Read the model definition and answer for the solid it produces. Units are mm, in the model's axes. A direction names the side the tool comes from. Coordinates: 2 decimals unless noted, no trailing zeros. Loops run counter-clockwise (first coordinate to the right, second up) from the corner with the lowest first, then second, coordinate; pieces in that order, holes last. Notation, with made-up numbers: (38, 83) -> (51, 83) arc R16 cw to (51, 100) -> close; hole circle Ø1 at (87, 54.25). An arc over 180 degrees is marked (long way). Answer as a JSON object with one key per item and string values. Group by question number.
Q1. The part is cut by section D-D on z = 8.5. Write down the section's boundary in (x, y).
Q2. The part is cut by section B-B on x = 12.5. State how many separate pieces and enclosed holes the cut face has, and give its area (3 significant figures).
Q3. Each of these flat-tipped pins is pushed along its axis until it touches: P1, Ø6, axis at y = 2, z = 5, coming from the +X side; P2, Ø1, axis at y = -3.5, z = 1, coming from the +X side; P3, Ø4, axis at x = -7, y = -2.5, coming from the -Z side; P4, Ø3, axis at y = 1.5, z = 1.5, coming from the -X side. Where does it stop, or does it pass through?
Q4. Straight lines are drawn through the part: line 1 along Y through (x, z) = (-13, 4.8); line 2 along Y through (x, z) = (12, 1.25); line 3 along Z through (x, y) = (-8.5, -4). For each, find the intervals that lie inside material, in ascending order. Write a range as [from, to].
Q5. The part is cut by section A-A on z = 5.25. Write down the section's boundary in (x, y), and give its area (3 significant figures).
Q6. Determine the mould class of faces 1 (the flat face through (7.5, 0, 5)), 2 (the cylindrical face through (18, 0, 9)), 3 (the flat face through (-10, 0, 7.5)) for opening direction Z: released by +Z, released by -Z, zero draft, split by the parting line, or undercut.
Q7. For faces 4 (the flat face through (10, 2, 2.2)), 5 (the flat face through (13, 3.05, 1)), 6 (the flat face through (-10, 0, 2.5)), 7 (the flat face through (-7.5, 0, 9)), determine the directions among +Z, -Z, +X, -X, +Y, -Y from which every point of the face is accessible in a straight line to the end or side of a thin tool.
from build123d import *

# Parameters (mm, degrees)
EXTRUDE_1_DEPTH     = 10
SKETCH_3_W          = 10.5
SKETCH_3_H          = 5.6
CUT_EXTRUDE_2_DEPTH = 23.891046285
SKETCH_4_W          = 10.5
SKETCH_4_H          = 2.5
CUT_EXTRUDE_3_DEPTH = 23.891046285
SKETCH_2_R          = 4
CUT_EXTRUDE_4_DEPTH = 3
CUT_EXTRUDE_4_DRAFT = -20
CUT_EXTRUDE_5_DEPTH = 2.5
SKETCH_9_R          = 2
CUT_EXTRUDE_8_DEPTH = 9


with BuildPart() as part:
    # Sketch 1 → Extrude 1 (new body)
    with BuildSketch(Plane.XY):
        with BuildLine():
            Line((-13, -5), (13, -5))
            ThreePointArc((13, -5), (18, 0), (13, 5))
            Line((13, 5), (-13, 5))
            ThreePointArc((-13, 5), (-18, 0), (-13, -5))
        make_face()
    extrude(amount=EXTRUDE_1_DEPTH)

    # Sketch 3 → Cut-Extrude 2 (cut, through all)
    with BuildSketch(Plane(origin=(0, 5, 0), x_dir=(1, 0, 0), z_dir=(0, 1, 0))):
        with Locations((12.75, -5)):
            Rectangle(SKETCH_3_W, SKETCH_3_H)
    extrude(amount=-CUT_EXTRUDE_2_DEPTH, mode=Mode.SUBTRACT)

    # Sketch 4 → Cut-Extrude 3 (cut, through all)
    with BuildSketch(Plane(origin=(0, 5, 0), x_dir=(1, 0, 0), z_dir=(0, 1, 0))):
        with Locations((-12.75, -1.25)):
            Rectangle(SKETCH_4_W, SKETCH_4_H)
        with Locations((-12.75, -8.75)):
            Rectangle(SKETCH_4_W, SKETCH_4_H)
    extrude(amount=-CUT_EXTRUDE_3_DEPTH, mode=Mode.SUBTRACT)


with BuildPart() as cut_extrude_4_tool:
    # Sketch 2 → Cut-Extrude 4 (with draft: the straight prism first)
    with BuildSketch(Plane.XY.offset(10)):
        with Locations((13, 0)):
            Circle(SKETCH_2_R)
    extrude(amount=-CUT_EXTRUDE_4_DEPTH)
    # Cut-Extrude 4: the draft: its side faces are tilted about the plane it starts from
    cut_extrude_4_sides = [cut_extrude_4_tool.faces().sort_by_distance(p)[0] for p in [
        (9, 0, 8.5),
    ]]
    draft(cut_extrude_4_sides, Plane.XY.offset(10), CUT_EXTRUDE_4_DRAFT)


with BuildPart() as part_1:
    add(part.part)

    # Cut-Extrude 4: cut by cut_extrude_4_tool
    add(cut_extrude_4_tool.part, mode=Mode.SUBTRACT)

    # Sketch 5 → Cut-Extrude 5 (cut)
    with BuildSketch(Plane(origin=(0, 0, 0), x_dir=(-1, 0, 0), z_dir=(0, 0, -1))):
        Polygon((-16.521836642, 0), (-14.760918321, -3.05), (-11.239081679, -3.05), (-9.478163358, 0), (-11.239081679, 3.05), (-14.760918321, 3.05), align=None)
    extrude(amount=-CUT_EXTRUDE_5_DEPTH, mode=Mode.SUBTRACT)

    # Sketch 9 → Cut-Extrude 8 (cut)
    with BuildSketch(Plane.XY):
        with Locations(Location((-13, 0, 0), (0, 0, 180))):
            Circle(SKETCH_9_R)
    extrude(amount=CUT_EXTRUDE_8_DEPTH, mode=Mode.SUBTRACT)


solid = part_1.part
Final values:
{
 "1": {"outline": "(-7.5, -5) -> (13, -5) arc R5 ccw to (13, 5) -> (-7.5, 5) -> close; hole circle Ø6.91 at (13, 0)"},
 "2": {"separate pieces": "4", "enclosed holes": "0", "area": "14.9 mm2"},
 "3": {"P1": "stops at x = 17.91", "P2": "stops at x = 17", "P3": "stops at z = 0", "P4": "stops at x = -17.99"},
 "4": {"line 1": "y = [-5, -2], [2, 5]", "line 2": "y = [-5, -3.05], [3.05, 5]", "line 3": "z = [2.5, 7.5]"},
 "5": {"outline": "(-13, -5) -> (7.5, -5) -> (7.5, 5) -> (-13, 5) arc R5 ccw to start; hole circle Ø4 at (-13, 0)", "area": "232 mm2"},
 "6": {"face 1": "undercut", "face 2": "zero draft", "face 3": "released by +Z"},
 "7": {"face 4": "+X, +Y, -Y", "face 5": "-Z", "face 6": "-Z, -X, +Y, -Y", "face 7": "+Z, -X, +Y, -Y"}
}
